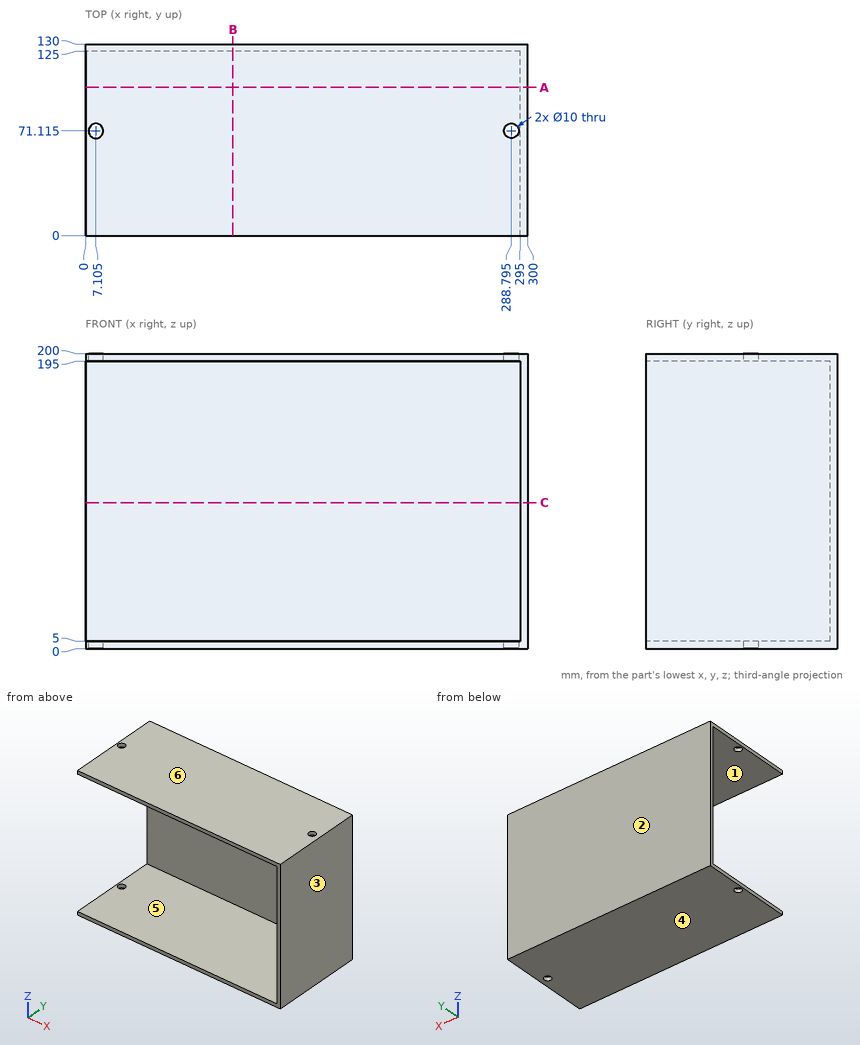
Geometry check sheet. Reference: drawing and pictorial views, mm from the part's lowest x, y, z. A direction names the side the tool comes from. Coordinates: 2 decimals unless noted, no trailing zeros. Order: outer loops, then holes, each group sorted by start corner. A loop starts at its lowest first (then second) coordinate and runs counter-clockwise, first axis right, second up. Notation, with made-up numbers: (13.25, 42) - (45.25, 42) arc R10 cw to (45.25, 60) - close; hole circle Ø8 at (57.25, 58.25). An arc over 180 degrees is marked (long way). Answer in a Markdown table with one row per item. Add a question column.
1) Cross-section at C-C, the plane z = 99. Record the cut outline in (x, y).
2) Release check for a two-part mould opening along Z. For the marked faces 3, 4, 5 and 6 record: +Z half, -Z half, draft (parallel to the pull), parting line (faces both ways), or undercut.
3) Cross-section at A-A, the plane y = 100.5. Record the cut outline in (x, z), then the cut area to 3 significant figures.
4) Cross-section at B-B, the plane x = 100. Record the cut outline in (y, z), then the cut area to 3 significant figures.
5) Material ranges on line 1 along Z through (x, y) = (54.5, 109.5); line 2 along Y through (x, z) = (227.5, 49.5); line 3 along X through (y, z) = (39, 55), recorded low to high. Write a range as [from, to].
6) Gauge pin test, flat ends, axial feed: P1, Ø12, axis at x = 116, z = 88, coming from the -Y side; P2, Ø10, axis at y = 35, z = 71, coming from the -X side. Record the tip position at first contact, or that the pin passes through.
7) Set-up check for the marked faces 1 and 2: record each of +Z, -Z, +X, -X, +Y, -Y from which the full face is reachable in a straight line by a thin tool's end or side.
Check result:
| question | item | result |
|---|---|---|
| 1 | outline | (0, 125) - (295, 125) - (295, 0) - (300, 0) - (300, 130) - (0, 130) - close |
| 2 | face 3 | draft |
| 2 | face 4 | -Z half |
| 2 | face 5 | undercut |
| 2 | face 6 | +Z half |
| 3 | outline | (0, 0) - (300, 0) - (300, 200) - (0, 200) - (0, 195) - (295, 195) - (295, 5) - (0, 5) - close |
| 3 | area | 3,950 mm² |
| 4 | outline | (0, 0) - (130, 0) - (130, 200) - (0, 200) - (0, 195) - (125, 195) - (125, 5) - (0, 5) - close |
| 4 | area | 2,250 mm² |
| 5 | line 1 | z = [0, 5], [195, 200] |
| 5 | line 2 | y = [125, 130] |
| 5 | line 3 | x = [295, 300] |
| 6 | P1 | stops at y = 125 |
| 6 | P2 | stops at x = 295 |
| 7 | face 1 | -X, -Y |
| 7 | face 2 | +Z, -Z, +X, -X, +Y |
